from build123d import *

# Parameters (mm, degrees)
CROQUIS1_R              = 70
CROQUIS1_R_2            = 5.5
SALIENTE_EXTRUIR1_DEPTH = 3


with BuildPart() as part:
    # Croquis1 → Saliente-Extruir1 (new body)
    with BuildSketch(Plane(origin=(0, 0, 0), x_dir=(1, 0, 0), z_dir=(0, 1, 0))):
        with Locations(Location((0, 0, 0), (0, 0, 270))):
            Circle(CROQUIS1_R)
        with Locations(Location((0, 0, 0), (0, 0, 270))):
            Circle(CROQUIS1_R_2, mode=Mode.SUBTRACT)
        Polygon((24.748737342, 24.748737342), (29.69848481, 19.798989873), (31.819805153, 21.920310217), (21.920310217, 31.819805153), (19.798989873, 29.69848481), align=None, mode=Mode.SUBTRACT)
        Polygon((24.748737342, -24.748737342), (19.798989873, -29.69848481), (21.920310217, -31.819805153), (31.819805153, -21.920310217), (29.69848481, -19.798989873), align=None, mode=Mode.SUBTRACT)
        Polygon((-24.748737342, 24.748737342), (-19.798989873, 29.69848481), (-21.920310217, 31.819805153), (-31.819805153, 21.920310217), (-29.69848481, 19.798989873), align=None, mode=Mode.SUBTRACT)
        Polygon((-24.748737342, -24.748737342), (-29.69848481, -19.798989873), (-31.819805153, -21.920310217), (-21.920310217, -31.819805153), (-19.798989873, -29.69848481), align=None, mode=Mode.SUBTRACT)
        Polygon((-14, 0), (-14, 9), (-17, 9), (-17, -9), (-14, -9), align=None, mode=Mode.SUBTRACT)
        Polygon((14, 0), (14, -9), (17, -9), (17, 9), (14, 9), align=None, mode=Mode.SUBTRACT)
        Polygon((0, -14), (-9, -14), (-9, -17), (9, -17), (9, -14), align=None, mode=Mode.SUBTRACT)
        Polygon((0, 62), (20, 62), (20, 59), (-20, 59), (-20, 62), align=None, mode=Mode.SUBTRACT)
        Polygon((55.861435714, 27.577164466), (27.577164466, 55.861435714), (29.69848481, 57.982756057), (43.840620434, 43.840620434), (57.982756057, 29.69848481), align=None, mode=Mode.SUBTRACT)
        Polygon((59, -20), (59, 20), (62, 20), (62, 0), (62, -20), align=None, mode=Mode.SUBTRACT)
        Polygon((27.577164466, -55.861435714), (55.861435714, -27.577164466), (57.982756057, -29.69848481), (43.840620434, -43.840620434), (29.69848481, -57.982756057), align=None, mode=Mode.SUBTRACT)
        Polygon((-20, -59), (20, -59), (20, -62), (0, -62), (-20, -62), align=None, mode=Mode.SUBTRACT)
        Polygon((-55.861435714, -27.577164466), (-27.577164466, -55.861435714), (-29.69848481, -57.982756057), (-43.840620434, -43.840620434), (-57.982756057, -29.69848481), align=None, mode=Mode.SUBTRACT)
        Polygon((-59, 20), (-59, -20), (-62, -20), (-62, 0), (-62, 20), align=None, mode=Mode.SUBTRACT)
        Polygon((-27.577164466, 55.861435714), (-55.861435714, 27.577164466), (-57.982756057, 29.69848481), (-43.840620434, 43.840620434), (-29.69848481, 57.982756057), align=None, mode=Mode.SUBTRACT)
    extrude(amount=SALIENTE_EXTRUIR1_DEPTH)


solid = part.part
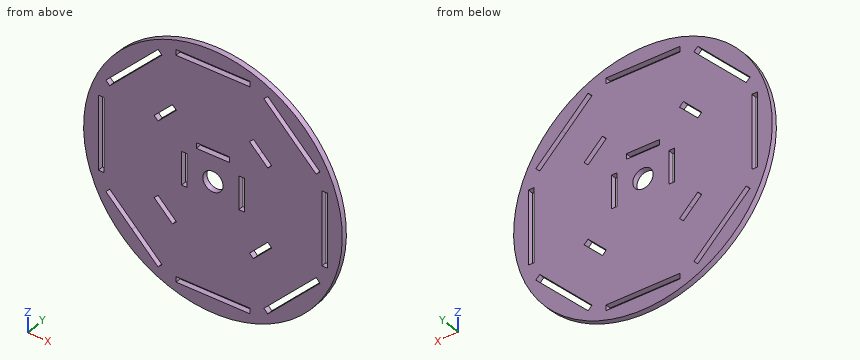
Geometry check sheet. Reference: the model listing, model coordinates, mm. Give positions to 0.01 mm unless a question says otherwise; leave off trailing zeros. Order: outer loops, then holes, each group sorted by start corner. A loop starts at its lowest first (then second) coordinate and runs counter-clockwise, first axis right, second up. Notation, with made-up numbers: (-10.75, -2.5) - (39.25, -2.5) arc R8 cw to (39.25, 5.5) - close; hole circle Ø6 at (42.25, -31). An arc over 180 degrees is marked (long way). Use one line per item in the form item = value.
1) Sectioned sample at B-B (x = 0). Record the boundary of the cut face in (y, z).
Working result:
outline = (0, -70) - (3, -70) - (3, -62) - (0, -62) - close; (0, -59) - (3, -59) - (3, -5.5) - (0, -5.5) - close; (0, 5.5) - (3, 5.5) - (3, 14) - (0, 14) - close; (0, 17) - (3, 17) - (3, 59) - (0, 59) - close; (0, 62) - (3, 62) - (3, 70) - (0, 70) - close
2) Sectioned sample at A-A (z = 0). Record the boundary of the cut face in (x, y).
Working result:
outline = (-70, 0) - (-62, 0) - (-62, 3) - (-70, 3) - close; (-59, 0) - (-17, 0) - (-17, 3) - (-59, 3) - close; (-14, 0) - (-5.5, 0) - (-5.5, 3) - (-14, 3) - close; (5.5, 0) - (14, 0) - (14, 3) - (5.5, 3) - close; (17, 0) - (59, 0) - (59, 3) - (17, 3) - close; (62, 0) - (70, 0) - (70, 3) - (62, 3) - close
3) Sectioned sample at C-C (z = 35). Record the boundary of the cut face in (x, y), and give its area (3 significant figures).
Working result:
outline = (-60.62, 0) - (-52.68, 0) - (-52.68, 3) - (-60.62, 3) - close; (-48.44, 0) - (48.44, 0) - (48.44, 3) - (-48.44, 3) - close; (52.68, 0) - (60.62, 0) - (60.62, 3) - (52.68, 3) - close
area = 338 mm^2
4) Depth check by flat-ended pin: pin 1 Ø0.9 at (y, z) = (1, 60.5) entering from -X; pin 2 Ø1.5 at (x, y) = (55, 1) entering from -Z; pin 3 Ø1.5 at (x, y) = (-3.5, 1.5) entering from -Z. Enter the tip coordinate at first touch or a pass-through.
Working result:
pin_1 = -35.97
pin_2 = -44.24
pin_3 = -69.95
5) Sectioned sample at D-D (y = 2.5). Count the separate pieces of the cut face and the enclosed holes in it, and give its area (3 significant figures).
Working result:
separate_pieces = 1
enclosed_holes = 16
area = 14,000 mm^2
6) Material ranges on probe 1 along X at (y, z) = (0.6, 0); probe 2 along X at (y, z) = (1, -54); probe 3 along X at (y, z) = (1.95, -23.5), recorded low to high. Write a range as from..to.
Working result:
probe_1 = -70..-62, -59..-17, -14..-5.5, 5.5..14, 17..59, 62..70
probe_2 = -44.54..-33.68, -29.44..29.44, 33.68..44.54
probe_3 = -65.94..-30.24, -26..26, 30.24..65.94
